from build123d import *

# Parameters (mm, degrees)
SKETCH_1_W = 4.5
SKETCH_1_H = 3


with BuildPart() as part:
    # Эскиз1 → Повернуть1 (revolve)
    with BuildSketch(Plane.XY, mode=Mode.PRIVATE) as revolve_1_sk:
        with BuildLine():
            Line((2.59417268, 8.339144345), (3.553438332, 5.67828869))
            ThreePointArc((3.553438332, 5.67828869), (3.308517433, 3.85034296), (1.671969637, 3))
            Line((1.671969637, 3), (-2.565092972, 3))
            ThreePointArc((-2.565092972, 3), (-4.201640768, 3.85034296), (-4.446561668, 5.67828869))
            Line((-4.446561668, 5.67828869), (-3.487296015, 8.339144345))
            ThreePointArc((-3.487296015, 8.339144345), (-3.121390188, 8.818273898), (-2.546561668, 9))
            Line((-2.546561668, 9), (1.653438332, 9))
            ThreePointArc((1.653438332, 9), (2.228266853, 8.818273898), (2.59417268, 8.339144345))
        make_face()
        with Locations((-0.446561668, 6.5)):
            Rectangle(SKETCH_1_W, SKETCH_1_H, mode=Mode.SUBTRACT)
    revolve(revolve_1_sk.sketch.rotate(Axis((-29.711247444, 0, 0), (1, 0, 0)), 90), axis=Axis((-29.711247444, 0, 0), (1, 0, 0)))


solid = part.part
Work out the finished part from the listing and answer in its coordinate system (mm). A direction names the side the tool comes from. Round coordinates to 2 decimals unless told otherwise and drop trailing zeros. Order: outer loops, then holes, each group sorted by start corner. A loop starts at its lowest first (then second) coordinate and runs counter-clockwise, first axis right, second up. Notation, with made-up numbers: M 13.5,-20 L 38.5,-20 A18 ccw 38.5,7 Z; hole C 86,33.5 d10. An arc over 180 degrees is marked long. Put each result on its own line as item: value. Start each with the question number.
Q1. Flat-ended cylindrical pins translate along their axes: pin 1 (1.5 mm diameter, centred on y = 5, z = -3.5, fed in from -X); pin 2 (3 mm diameter, centred on x = -2, y = 2.5, fed in from -Z); pin 3 (2 mm diameter, centred on x = -1, y = 4, fed in from +Z). Find the tip coordinate at first contact, or state that the pin passes through.
Q2. For a pull along Z with two mould halves and no side action, classify faces 1 (the cylindrical face through (-0.417, -6.083, -6.633)), 2 (the cylindrical face through (-0.42, 7.81, -1.73)), 3 (the flat face through (-2.697, -0.1, -5.2)) as pulls with the +Z half, pulls with the -Z half, needs draft (parallel to the pull), parting line crosses it, or undercut.
Q3. A tool of negligible diameter and unlimited length cuts with its end or side. For faces 4 (the cylindrical face through (0, 0, -5)), 5 (the conical face through (-4.387, 5.706, -1.267)), from which of +Z, -Z, +X, -X, +Y, -Y can it reach the whole face along a straight path? Write none if from no direction.
Q4. Straight lines are drawn through the part: L1, parallel to Y at x = -0.9, z = 0; L2, parallel to Z at x = 1, y = -1.75; L3, parallel to Y at x = 0.25, z = 4.25. For each, find the intervals that lie inside material, in ascending order. Write a range as [from, to].
Q5. Section C-C, the plane x = -1 is taken. Write down the section's boundary in (y, z).
Q6. Section D-D, the plane z = -4 is taken. Give the number of separate pieces and of enclosed holes in the cut face, and give its area (3 significant figures).
Q7. Section A-A, the plane y = 0 is taken. Write down the section's boundary in (x, z), and give its area (3 significant figures).
Findings below:
1. pin 1: stops at x = -4.53
1. pin 2: stops at z = -8.94
1. pin 3: stops at z = 8.49
2. face 1: parting line crosses it
2. face 2: undercut
2. face 3: undercut
3. face 4: none
3. face 5: -X
4. L1: y = [-9, -8], [-5, -3], [3, 5], [8, 9]
4. L2: z = [-8.83, -7.81], [-4.68, -2.44], [2.44, 4.68], [7.81, 8.83]
4. L3: y = [-7.93, -6.78], [-2.63, 2.63], [6.78, 7.93]
5. outline: C 0,0 d18; C 0,0 d10; hole C 0,0 d16; hole C 0,0 d6
6. separate pieces: 1
6. enclosed holes: 2
6. area: 84.1 mm^2
7. outline: M -4.45,-5.68 L -3.49,-8.34 A1 ccw -2.55,-9 L 1.65,-9 A1 ccw 2.59,-8.34 L 3.55,-5.68 A2 ccw 1.67,-3 L -2.57,-3 A2 ccw Z; M -4.45,5.68 A2 ccw -2.57,3 L 1.67,3 A2 ccw 3.55,5.68 L 2.59,8.34 A1 ccw 1.65,9 L -2.55,9 A1 ccw -3.49,8.34 Z; hole M -2.7,-8 L 1.8,-8 L 1.8,-5 L -2.7,-5 Z; hole M -2.7,5 L 1.8,5 L 1.8,8 L -2.7,8 Z
7. area: 58.4 mm^2
